Autodesk Inventor part; units mm, degrees
ref_plane "YZ Plane" through (0, 0, 0) normal (1, 0, 0) x (0, 1, 0)
ref_plane "XZ Plane" through (0, 0, 0) normal (0, 1, 0) x (-1, 0, 0)
ref_plane "XY Plane" through (0, 0, 0) normal (0, 0, 1) x (1, 0, 0)
sketch "Sketch1" plane through (0, 0, 0) normal (0, 0, 1) x (1, 0, 0)
  line L0 (-26, 5) -> (26, 5)
  line L1 (26, 5) -> (26, -5)
  line L2 (26, -5) -> (-26, -5)
  line L3 (-26, -5) -> (-26, 5)
  point P0 (0, 0)
  dimension "d0" = 52
  dimension "d1" = 10
extrude "Extrusion1" add sketch "Sketch1" along normal blind 1.5
sketch "Sketch2" plane through (-26, -5, 0) normal (0, -1, 0) x (1, 0, 0)
  line L0 (0, 1.5) -> (52, 1.5)
  line L1 (26, 1.5) -> (13, 1.5)
  line L2 (13, 4.7) -> (15, 4.7)
  line L3 (15, 4.7) -> (15, 1.5)
  line L4 (13, 4.7) -> (13, 6.3)
  line L5 (13, 6.3) -> (15, 8.3)
  line L6 (13, 6.3) -> (15.8284, 6.3) construction
  line L7 (15, 8.3) -> (11, 8.3)
  line L8 (11, 8.3) -> (11, 1.5)
  line L9 (52, 1.5) -> (0, 1.5)
  line L10 (11, 1.5) -> (15, 1.5)
  line L11 (26, 1.5) -> (26, 4.9)
  line L12 (39, 4.7) -> (37, 4.7)
  line L13 (37, 4.7) -> (37, 1.5)
  line L14 (39, 4.7) -> (39, 6.3)
  line L15 (39, 6.3) -> (37, 8.3)
  line L16 (39, 6.3) -> (36.1716, 6.3) construction
  line L17 (37, 8.3) -> (41, 8.3)
  line L18 (41, 8.3) -> (41, 1.5)
  line L19 (41, 1.5) -> (37, 1.5)
  point P0 (26, 0)
  point P1 (39, 1.5)
  dimension "d4" = 13
  dimension "d5" = 3.2
  dimension "d6" = 2
  dimension "d7" = 1.6
  dimension "d8" = 45
extrude "Extrusion2" add sketch "Sketch2" against normal blind 10
sketch "Sketch3" plane through (-26, -5, 0) normal (0, -1, 0) x (1, 0, 0)
  line L0 (0, 0) -> (52, 0)
  line L1 (0, 0) -> (0, -1.5)
  line L2 (0, 0) -> (0, 1.5)
  line L3 (0, 1.5) -> (-1.5, 1.5)
  line L4 (0, -1.5) -> (0.75, -2.25)
  line L5 (0, -1.5) -> (4.2622, -1.5) construction
  line L6 (0.75, -2.25) -> (-0.3107, -3.3107)
  line L7 (0.75, -2.25) -> (-0.3107, -3.3107)
  line L8 (0, 1.5) -> (-1.5, 1.5)
  line L9 (-1.5, 1.5) -> (-1.5, -2.1213)
  line L10 (-0.3107, -3.3107) -> (-1.5, -2.1213)
  line L11 (26, 0) -> (26, -3.3107)
  line L12 (52, 0) -> (52, -1.5)
  line L13 (52, 0) -> (52, 1.5)
  line L14 (52, 1.5) -> (53.5, 1.5)
  line L15 (52, -1.5) -> (51.25, -2.25)
  line L16 (52, -1.5) -> (47.7378, -1.5) construction
  line L17 (51.25, -2.25) -> (52.3107, -3.3107)
  line L18 (51.25, -2.25) -> (52.3107, -3.3107)
  line L19 (52, 1.5) -> (53.5, 1.5)
  line L20 (53.5, 1.5) -> (53.5, -2.1213)
  line L21 (52.3107, -3.3107) -> (53.5, -2.1213)
  dimension "d11" = 1.5
  dimension "d13" = 45
  dimension "d15" = 1.5
extrude "Extrusion3" add sketch "Sketch3" against normal blind 10
fillet "Fillet1" radius 0.5 4 edges at (-25.25, 0, -2.25) (-26.3107, 0, -3.3107) (25.25, 0, -2.25) (26.3107, 0, -3.3107)
fillet "Fillet2" radius 1 2 edges at (-15, 0, 8.3) (15, 0, 8.3)
fillet "Fillet3" radius 0.5 2 edges at (-11, 0, 8.3) (11, 0, 8.3)
fillet "Fillet4" radius 0.5 2 edges at (-11, 0, 4.7) (11, 0, 4.7)
properties part number "env_combo_holder"
Design review of the part built by this model. Coordinates are the model's own, in mm. A direction names the side the tool comes from. Give positions to 0.01 mm unless a question says otherwise; leave off trailing zeros. Order: outer loops, then holes, each group sorted by start corner. A loop starts at its lowest first (then second) coordinate and runs counter-clockwise, first axis right, second up. Notation, with made-up numbers: (8.25, 23) -> (16.25, 23) arc R30 ccw to (16.25, 51) -> close; hole circle Ø5 at (-6, -19.75). An arc over 180 degrees is marked (long way). Write each question's results on one line, items separated by ' | '. Start each with the question number.
Q1. Machinability: for faces 4 (the flat face through (15, 0, 4)), 5 (the flat face through (-15, 0, 4)), 6 (the flat face through (-11, 0, 3)), 7 (the flat face through (-13, 0, 5)), which of the approach directions +Z, -Z, +X, -X, +Y, -Y give a long, thin tool a straight path to every point of the face, cutting with its end or side? Answer none if there is none.
Q2. Wall thickness on L1, parallel to X at y = 4.25, z = 2; L2, parallel to X at y = -1.5, z = -0.75; L3, parallel to Z at x = -17.5, y = -3.5: over which ranges is each line inside the solid? List them lowest first. Write a range as from..to.
Q3. For pin 1 (5 mm diameter, centred on x = 12.5, z = -2, fed in from +Y); pin 2 (1.7 mm diameter, centred on y = 0, z = 4, fed in from -X); pin 3 (3 mm diameter, centred on x = 9, y = 3.5, fed in from +Z); pin 4 (0.5 mm diameter, centred on y = 0, z = 5.5, fed in from +X), all flat-tipped, find the tip position at first contact; note any pin that passes through.
Q4. Mouldability with a two-part tool opening along Z and no side actions: class faces 1 (the flat face through (21, 0, 1.5)), 2 (the flat face through (13, 0, 5)), 3 (the flat face through (27.5, 0, 0)) as +Z half, -Z half, draft (parallel to the pull), parting line (faces both ways), or undercut.
Q5. Add section A-A on z = 3. Give the boundary of the cut face in (x, y).
Q6. Add section B-B on x = 17. Give the boundary of the cut face in (y, z), and give its area (3 significant figures).
Found:
1) face 4: +Z, +X, +Y, -Y | face 5: +Z, -X, +Y, -Y | face 6: +Z, +Y, -Y | face 7: +Y, -Y
2) L1: x = -15..-11, 11..15 | L2: x = -27.5..-26, 26..27.5 | L3: z = 0..1.5
3) pin 1: stops at y = 5 | pin 2: stops at x = -15 | pin 3: stops at z = 1.5 | pin 4: stops at x = 15
4) face 1: +Z half | face 2: undercut | face 3: draft
5) outline: (-15, -5) -> (-11, -5) -> (-11, 5) -> (-15, 5) -> close; (11, -5) -> (15, -5) -> (15, 5) -> (11, 5) -> close
6) outline: (-5, 0) -> (5, 0) -> (5, 1.5) -> (-5, 1.5) -> close | area: 15.0 mm2
